Input: dimensioned drawing with shaded views. Units: mm. Origin: part minimum x, y, z. A direction names the side the tool comes from. Coordinates: 2 decimals unless noted, no trailing zeros. Order: outer loops, then holes, each group sorted by start corner. A loop starts at its lowest first (then second) coordinate and runs counter-clockwise, first axis right, second up.
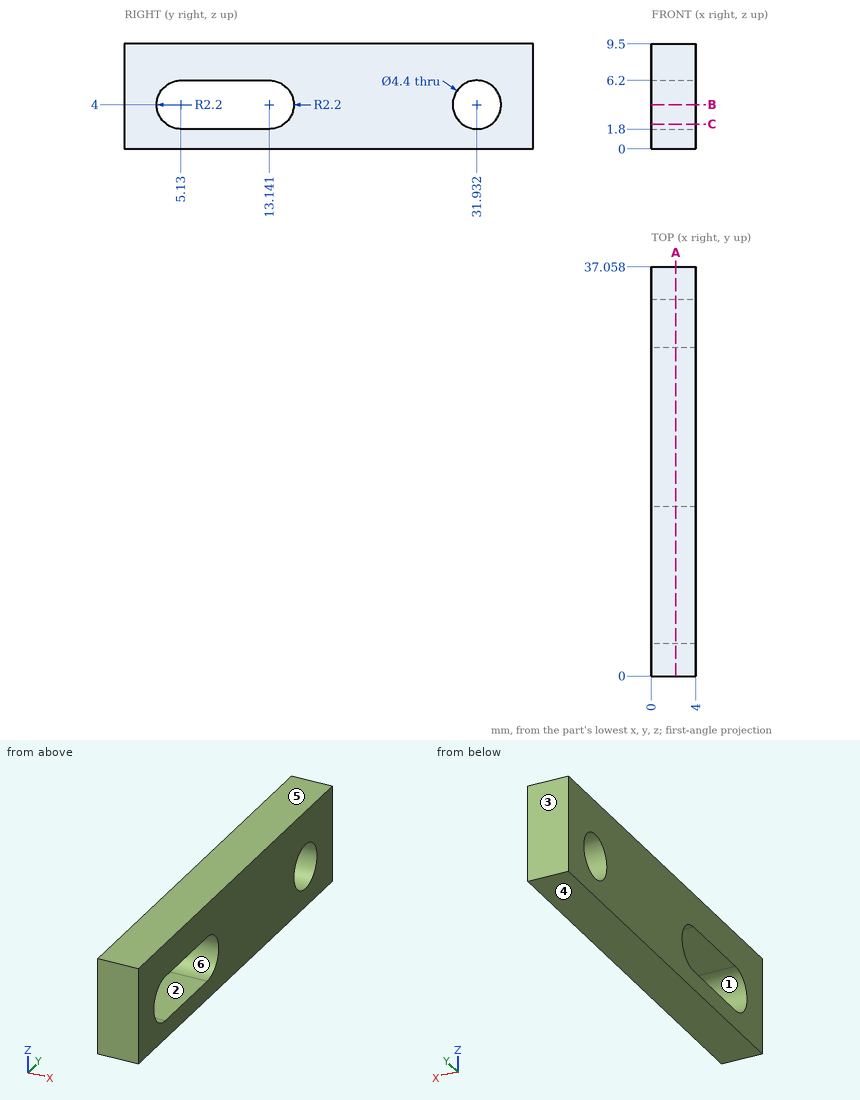
1. Draft query along Y for the marked faces 1, 2, 3 and 4. Return one class per face: released by +Y, released by -Y, zero draft, split by the parting line, or undercut.
Findings:
face 1: undercut
face 2: undercut
face 3: released by +Y
face 4: zero draft
2. Access query for the marked faces 5 and 6. Directions: +Z, -Z, +X, -X, +Y, -Y. A direction counts if a zero-diameter tool reaches every point of the face in a straight line with its end or side. Return the directions, or none.
Findings:
face 5: +Z, +X, -X, +Y, -Y
face 6: +X, -X
3. Section query B-B on z = 4. Return loops of the section in (x, y).
Findings:
outline: (0, 0) - (4, 0) - (4, 2.93) - (0, 2.93) - close; (0, 15.34) - (4, 15.34) - (4, 29.73) - (0, 29.73) - close; (0, 34.13) - (4, 34.13) - (4, 37.06) - (0, 37.06) - close
4. Pin query (flat end, axial travel): P1, Ø1.5, axis at x = 1, z = 1.5, coming from the -Y side. Return the tip coordinate at first contact, or that it passes through.
Findings:
P1: stops at y = 0
5. Section query A-A on x = 2.2. Return loops of the section in (y, z).
Findings:
outline: (0, 0) - (37.06, 0) - (37.06, 9.5) - (0, 9.5) - close; hole (5.13, 1.8) - (13.14, 1.8) arc R2.2 ccw to (13.14, 6.2) - (5.13, 6.2) arc R2.2 ccw to start; hole circle Ø4.4 at (31.93, 4)
6. Ray query, line 1 (Z direction, x = 3.75, y = 6.5); line 2 (Z direction, x = 1.05, y = 32.5) (1 decimal). Return the intervals inside material, ascending.
Findings:
line 1: z = 0 to 1.8, 6.2 to 9.5
line 2: z = 0 to 1.9, 6.1 to 9.5
7. Section query C-C on z = 2.25. Return loops of the section in (x, y) (1 decimal).
Findings:
outline: (0, 0) - (4, 0) - (4, 3.8) - (0, 3.8) - close; (0, 14.5) - (4, 14.5) - (4, 30.6) - (0, 30.6) - close; (0, 33.3) - (4, 33.3) - (4, 37.1) - (0, 37.1) - close
